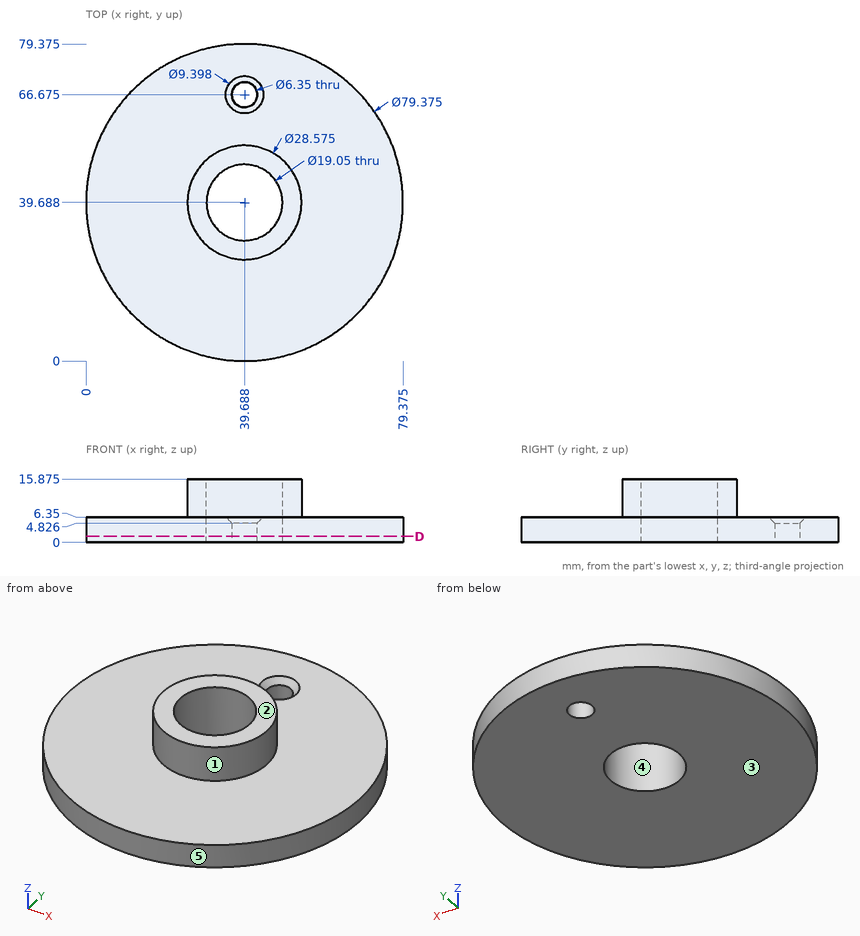
Design review of the part shown in the three views and the two pictorial views. Dimensions are in mm from the part's minimum x, y and z. A direction names the side the tool comes from. Round coordinates to 2 decimals unless told otherwise and drop trailing zeros. Answer as a JSON object with one key per item and string values.
1. To check wall thickness, follow line 1 along Z through (x, y) = (56, 53); line 2 along Y through (x, z) = (34, 2.5) (1 decimal); line 3 along X through (y, z) = (47, 4.25) (1 decimal). State the ranges of each line that lie inside material, in increasing order.
Results found:
{"line 1": "z = 0 to 6.35", "line 2": "y = 0.4 to 32, 47.3 to 79", "line 3": "x = 0.7 to 33.6, 45.8 to 78.7"}
2. The part is to be moulded in two halves that separate along Y. For the marked faces 3, 4 and 5, say which applies: pulls with the +Y half, pulls with the -Y half, needs draft (parallel to the pull), parting line crosses it, or undercut.
Results found:
{"face 3": "needs draft", "face 4": "undercut", "face 5": "parting line crosses it"}
3. We need section D-D on z = 1.5. State how many separate pieces and enclosed holes the cut face has, and give its area (3 significant figures).
Results found:
{"separate pieces": "1", "enclosed holes": "2", "area": "4,630 mm^2"}
4. Machinability: for the marked faces 1 and 2, which of the approach directions +Z, -Z, +X, -X, +Y, -Y give a long, thin tool a straight path to every point of the face, cutting with its end or side? Answer none if there is none.
Results found:
{"face 1": "+Z", "face 2": "+Z, +X, -X, +Y, -Y"}
5. Clearance check with flat-ended pins moving along their axes: pin 1 (5 mm diameter, centred on y = 27.5, z = 10, fed in from +X); pin 2 (8 mm diameter, centred on x = 52.5, z = 6.5, fed in from +Y); pin 3 (1.5 mm diameter, centred on x = 33.5, z = 9.5, fed in from +Y). State where each tip first meets the part, or that it passes through.
Results found:
{"pin 1": "stops at x = 50.19", "pin 2": "stops at y = 78.38", "pin 3": "stops at y = 52.9"}
